Verification items for the finished model (mm, model axes). Face numbers are marked on the shaded views. Give positions to 0.01 mm unless a question says otherwise; leave off trailing zeros. Write each question's results on one line, items separated by ' | '. Start each with the question number.
1. Depth check by flat-ended pin: pin 1 Ø2 at (x, z) = (-6, -8.5) entering from +Y; pin 2 Ø2 at (x, y) = (-0.5, 15) entering from +Z; pin 3 Ø10 at (x, y) = (-10, 4.5) entering from +Z. Enter the tip coordinate at first touch or a pass-through.
2. Material ranges on L1, parallel to Z at x = 0, y = 13.25; L2, parallel to Z at x = 3.5, y = 10.25, recorded low to high. Write a range as from..to.
3. Mould release check, pull along Z, two halves, no side actions. Record for the marked faces 1, 2 and 3: +Z half, -Z half, draft (parallel to the pull), parting line (faces both ways), or undercut.
from build123d import *

# Parameters (mm, degrees)
FILLET1_R = 2.5
FILLET2_R = 1


with BuildPart() as part:
    # Sketch1 → Revolve1 (revolve)
    with BuildSketch(Plane.XY):
        Polygon((6.35, 19.05), (7.14375, 19.05), (7.9375, 17.231027131), (7.9375, 5.08), (15, 2.54), (15, 0), (6.35, 0), align=None)
    revolve(axis=Axis((0, -0.9525, 0), (0, 1, 0)))

    # Fillet1
    fillet1_edges = [part.edges().sort_by_distance(p)[0] for p in [
        (-15, 2.54, 0),
    ]]
    fillet(fillet1_edges, radius=FILLET1_R)

    # Fillet2
    fillet2_edges = [part.edges().sort_by_distance(p)[0] for p in [
        (-7.9375, 5.08, 0),
    ]]
    fillet(fillet2_edges, radius=FILLET2_R)


solid = part.part
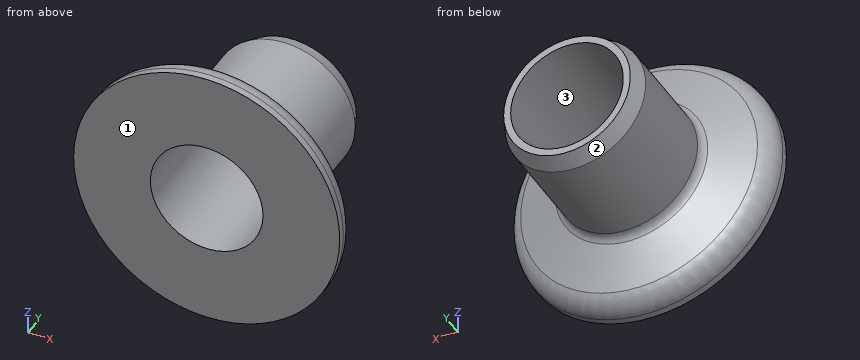
Results below:
1) pin 1: stops at y = 4.55 | pin 2: stops at z = 7.94 | pin 3: stops at z = 13.63
2) L1: z = -7.94..-6.35, 6.35..7.94 | L2: z = -7.12..-5.3, 5.3..7.12
3) face 1: draft | face 2: parting line | face 3: undercut
